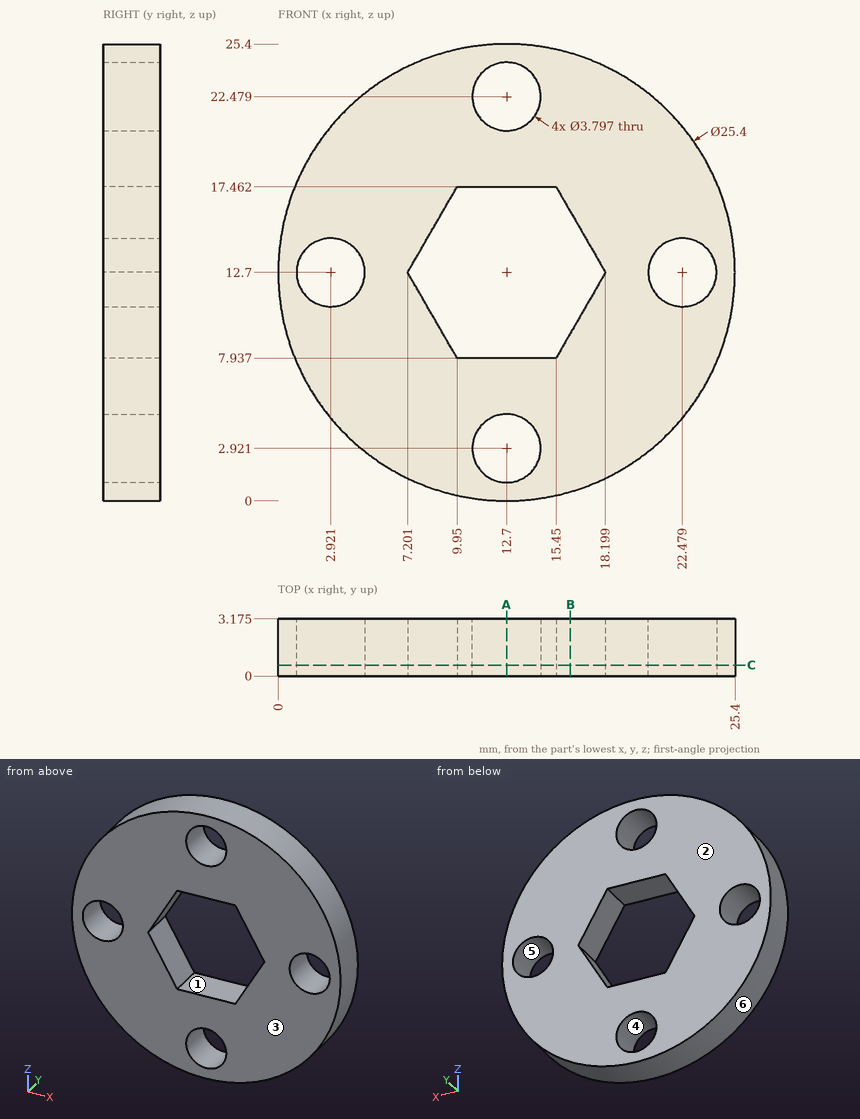
Check sheet for the drawn part. Datum: minimum x, y, z corner. Units: mm. A direction names the side the tool comes from. Give positions to 0.01 mm unless a question says otherwise; leave off trailing zeros. Loops run counter-clockwise (first coordinate to the right, second up) from the corner with the lowest first, then second, coordinate; pieces in that order, holes last.
1) Sectioned sample at B-B, the plane x = 16.25. Enter the section's corners in (y, z) (1 decimal).
2) Set-up check for the marked faces 1 and 2: record each of +Z, -Z, +X, -X, +Y, -Y from which the full face is reachable in a straight line by a thin tool's end or side.
3) Sectioned sample at C-C, the plane y = 0.6. Enter the section's corners in (x, z).
4) Thickness scan on line 1 along Z through (x, y) = (12.7, 1.2); line 2 along X through (y, z) = (0.9, 9.25); line 3 along Z through (x, y) = (2.25, 2.6) (1 decimal). Record the ranges inside material, lowest first.
5) Sectioned sample at A-A, the plane x = 12.7. Enter the section's corners in (y, z) (1 decimal).
6) Depth check by flat-ended pin: pin 1 Ø1.5 at (x, y) = (7, 2) entering from -Z (1 decimal); pin 2 Ø1.5 at (y, z) = (2, 8.5) entering from +X; pin 3 Ø6 at (x, z) = (12.7, 22.479) entering from -Y. Enter the tip coordinate at first touch or a pass-through.
7) Draft check along X on the marked faces 3, 4, 5 and 6. Enter one of: pulls with the +X half, pulls with the -X half, needs draft (parallel to the pull), parting line crosses it, or undercut.
Answers:
1. outline: (0, 0.5) - (3.2, 0.5) - (3.2, 9.3) - (0, 9.3) - close; (0, 16.1) - (3.2, 16.1) - (3.2, 24.9) - (0, 24.9) - close
2. face 1: +Y, -Y
2. face 2: +Z, -Z, +X, -X, +Y
3. outline: circle Ø25.4 at (12.7, 12.7); hole circle Ø3.8 at (2.92, 12.7); hole (7.2, 12.7) - (9.95, 7.94) - (15.45, 7.94) - (18.2, 12.7) - (15.45, 17.46) - (9.95, 17.46) - close; hole circle Ø3.8 at (12.7, 2.92); hole circle Ø3.8 at (12.7, 22.48); hole circle Ø3.8 at (22.48, 12.7)
4. line 1: z = 0 to 1.02, 4.82 to 7.94, 17.46 to 20.58, 24.38 to 25.4
4. line 2: x = 0.48 to 9.19, 16.21 to 24.92
4. line 3: z = 5.5 to 10.9, 14.5 to 19.9
5. outline: (0, 0) - (3.2, 0) - (3.2, 1) - (0, 1) - close; (0, 4.8) - (3.2, 4.8) - (3.2, 7.9) - (0, 7.9) - close; (0, 17.5) - (3.2, 17.5) - (3.2, 20.6) - (0, 20.6) - close; (0, 24.4) - (3.2, 24.4) - (3.2, 25.4) - (0, 25.4) - close
6. pin 1: stops at z = 1
6. pin 2: stops at x = 24.92
6. pin 3: stops at y = 0
7. face 3: needs draft
7. face 4: undercut
7. face 5: undercut
7. face 6: parting line crosses it
